from build123d import *

# Parameters (mm, degrees)
F1_DEPTH = 19.05


with BuildPart() as f1:
    # F0 (on Top) → F1 (new body)
    with BuildSketch(Plane.XY):
        Polygon((297.050197, 397.317676), (-109.349803, 397.317676), (-109.349803, -466.282324), (-58.057822, -466.282324), (178.001612, -399.338305), (237.651035, -466.282324), (297.050197, -466.282324), align=None)
        Polygon((-28.267516, -225.826263), (-25.87169, -26.973946), (211.31359, -221.034646), align=None, mode=Mode.SUBTRACT)
        Polygon((228.767082, 46.128679), (223.69054, -113.782555), (-39.020769, 25.82249), align=None, mode=Mode.SUBTRACT)
        Polygon((-2.2158, 227.615237), (243.996739, 75.318821), (-40.289905, 88.010184), align=None, mode=Mode.SUBTRACT)
    extrude(amount=F1_DEPTH)


solid = f1.part
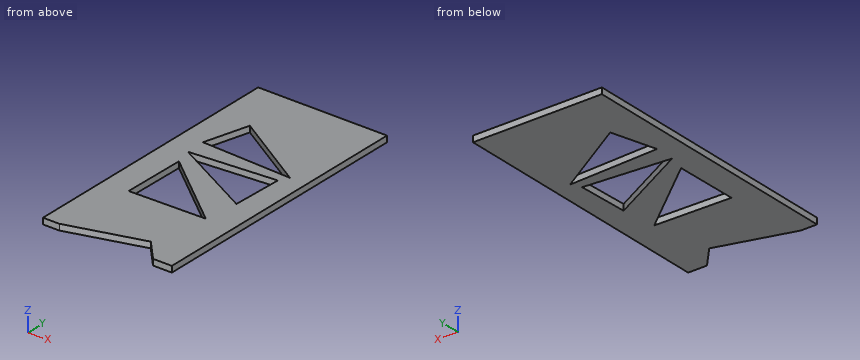
Geometry check sheet. Reference: the model listing, model coordinates, mm. Round coordinates to 2 decimals unless told otherwise and drop trailing zeros. Write each loop counter-clockwise with the first axis right and the second up, starting at its lowest first coordinate (ties: lowest second). Pieces come first, ordered by that corner, then holes.
Item 1: Section check B-B (y = -181). Record the boundary of the cut face in (x, z).
Determined:
outline: (-109.35, 0) - (-27.73, 0) - (-27.73, 19.05) - (-109.35, 19.05) - close; (162.38, 0) - (297.05, 0) - (297.05, 19.05) - (162.38, 19.05) - close
Item 2: Material ranges on line 1 along Y through (x, z) = (160.5, 11); line 2 along Y through (x, z) = (207.5, 7.5); line 3 along X through (y, z) = (-155, 18), recorded low to high.
Determined:
line 1: y = -404.3 to -222.05, -179.46 to -80.2, 40.95 to 79.05, 126.97 to 397.32
line 2: y = -432.44 to -221.11, -217.91 to -105.18, 44.52 to 76.95, 97.89 to 397.32
line 3: x = -109.35 to -27.41, 130.6 to 297.05
Item 3: Section check C-C (x = 27.5). Record the boundary of the cut face in (y, z).
Determined:
outline: (-442.02, 0) - (-224.71, 0) - (-224.71, 19.05) - (-442.02, 19.05) - close; (-70.64, 0) - (-9.53, 0) - (-9.53, 19.05) - (-70.64, 19.05) - close; (30.87, 0) - (84.98, 0) - (84.98, 19.05) - (30.87, 19.05) - close; (209.23, 0) - (397.32, 0) - (397.32, 19.05) - (209.23, 19.05) - close
Item 4: Section check D-D (y = -57). Record the boundary of the cut face in (x, z).
Determined:
outline: (-109.35, 0) - (-26.23, 0) - (-26.23, 19.05) - (-109.35, 19.05) - close; (10.83, 0) - (116.84, 0) - (116.84, 19.05) - (10.83, 19.05) - close; (225.49, 0) - (297.05, 0) - (297.05, 19.05) - (225.49, 19.05) - close
Item 5: Section check A-A (z = 4). Record the boundary of the cut face in (x, y).
Determined:
outline: (-109.35, -466.28) - (-58.06, -466.28) - (178, -399.34) - (237.65, -466.28) - (297.05, -466.28) - (297.05, 397.32) - (-109.35, 397.32) - close; hole (-40.29, 88.01) - (244, 75.32) - (-2.22, 227.62) - close; hole (-39.02, 25.82) - (223.69, -113.78) - (228.77, 46.13) - close; hole (-28.27, -225.83) - (211.31, -221.03) - (-25.87, -26.97) - close
